from build123d import *

# Parameters (mm, degrees)
F0_W     = 50.8
F0_H     = 9.525
F1_DEPTH = 63.5
F2_R     = 3.175
F3_DEPTH = 9.525
F4_R     = 3.175
F5_DEPTH = 12.7
F6_R     = 5.08
F7_SIZE  = 1.27


# Not quite as in the source:
# - a length typed as a fraction of an inch, garbled in the dataset ("3 / 203.2 mm" for 3/8 in), is restored


with BuildPart() as f1:
    # F0 (on Top) → F1 (new body)
    with BuildSketch(Plane.XY):
        with Locations((-25.4, 4.7625)):
            Rectangle(F0_W, F0_H)
    extrude(amount=F1_DEPTH)

    # F2 (on face) → F3 (cut)
    with BuildSketch(Plane.XZ):
        with Locations((-25.4, 50.8)):
            Circle(F2_R)
    extrude(amount=-F3_DEPTH, mode=Mode.SUBTRACT)

    # F4 (on face) → F5 (cut)
    with BuildSketch(Plane(origin=(0, 0, 0), x_dir=(1, 0, 0), z_dir=(0, 0, -1))):
        with Locations((-38.1, -4.7625)):
            Circle(F4_R)
        with Locations((-12.7, -4.7625)):
            Circle(F4_R)
    extrude(amount=-F5_DEPTH, mode=Mode.SUBTRACT)

    # F6
    f6_edges = [f1.edges().sort_by_distance(p)[0] for p in [
        (-50.8, 4.7625, 63.5),
        (0, 4.7625, 63.5),
    ]]
    fillet(f6_edges, radius=F6_R)

    # F7
    f7_edges = [f1.edges().sort_by_distance(p)[0] for p in [
        (-28.575, 0, 50.8),
        (-28.575, 9.525, 50.8),
    ]]
    chamfer(f7_edges, length=F7_SIZE)


solid = f1.part
The listing builds one solid part. Answer for the finished solid, in the listing's coordinates (mm). A direction names the side the tool comes from. Round coordinates to 2 decimals unless told otherwise and drop trailing zeros. Write each loop counter-clockwise with the first axis right and the second up, starting at its lowest first coordinate (ties: lowest second). Pieces come first, ordered by that corner, then holes. Notation, with made-up numbers: M 2.25,9.25 L 12.25,9.25 A14 cw 12.25,34.25 Z; hole C 87.25,49 d6. An arc over 180 degrees is marked long. Write each question's results on one line, items separated by ' | '. Start each with the question number.
Item 1: A cutting plane is placed at B-B on z = 50.8. Write down the section's boundary in (x, y) (3 decimals).
Item 2: A cutting plane is placed at C-C on x = -12.7. Write down the section's boundary in (y, z) (1 decimal), and give its area (3 significant figures).
Item 3: A cutting plane is placed at D-D on y = 3.5. Write down the section's boundary in (x, z) (3 decimals).
Item 4: Flat-ended cylindrical pins translate along their axes: pin 1 Ø10 at (x, z) = (-27, 33.5) entering from -Y; pin 2 Ø5.5 at (x, z) = (-25.4, 50.8) entering from -Y. Find the tip coordinate at first contact, or state that the pin passes through.
Item 5: For a pull along X with two mould halves and no side action, classify faces 1 (the face through (-38, 5, 12.7)), 2 (the face through (-1.528, 4.829, 62.051)), 3 (the face through (-50.8, 5, 29)) as pulls with the +X half, pulls with the -X half, needs draft (parallel to the pull), parting line crosses it, or undercut.
Item 6: Straight lines are drawn through the part: L1, parallel to Y at x = -38, z = 7 (3 decimals); L2, parallel to Z at x = -25.4, y = 3 (3 decimals); L3, parallel to Z at x = -41, y = 5.5. For each, find the intervals that lie inside material, in ascending order. Write a range as [from, to].
Item 7: A cutting plane is placed at A-A on x = -25.4. Write down the section's boundary in (y, z) (3 decimals).
Item 8: For faces 4 (the face through (-26, 0, 31)), 5 (the face through (-13, 5, 12.7)), determine the directions among +Z, -Z, +X, -X, +Y, -Y from which every point of the face is accessible in a straight line to the end or side of a thin tool.
Check sheet entries:
1) outline: M -50.8,0 L -29.845,0 L -28.575,1.27 L -28.575,8.255 L -29.845,9.525 L -50.8,9.525 Z; M -22.225,1.27 L -20.955,0 L 0,0 L 0,9.525 L -20.955,9.525 L -22.225,8.255 Z
2) outline: M 0,0 L 1.6,0 L 1.6,12.7 L 7.9,12.7 L 7.9,0 L 9.5,0 L 9.5,63.5 L 0,63.5 Z | area: 524 mm²
3) outline: M -50.8,0 L -41.013,0 L -41.013,12.7 L -35.187,12.7 L -35.187,0 L -15.613,0 L -15.613,12.7 L -9.787,12.7 L -9.787,0 L 0,0 L 0,58.42 A5.08 ccw -5.08,63.5 L -45.72,63.5 A5.08 ccw -50.8,58.42 Z; hole C -25.4,50.8 d6.35
4) pin 1: y = 0 | pin 2: through
5) face 1: undercut | face 2: pulls with the +X half | face 3: pulls with the -X half
6) L1: [0, 1.589], [7.936, 9.525] | L2: [0, 47.625], [53.975, 63.5] | L3: [12.7, 63.5]
7) outline: M 0,0 L 9.525,0 L 9.525,46.355 L 8.255,47.625 L 1.27,47.625 L 0,46.355 Z; M 0,55.245 L 1.27,53.975 L 8.255,53.975 L 9.525,55.245 L 9.525,63.5 L 0,63.5 Z
8) face 4: +Z, -Z, +X, -X, -Y | face 5: -Z
